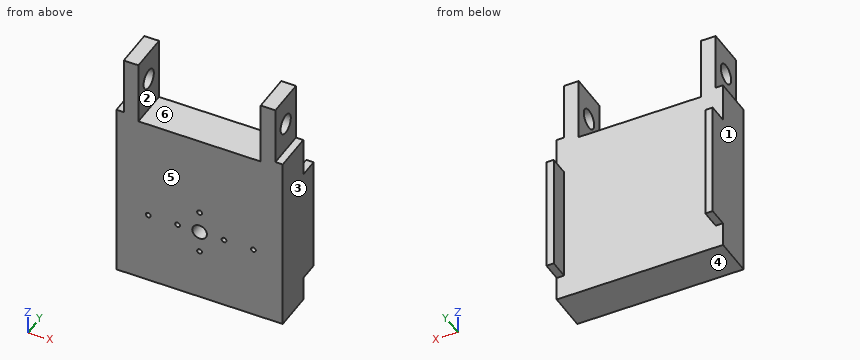
from build123d import *

# Parameters (mm, degrees)
SKETCH_1_W          = 34
SKETCH_1_H          = 49
EXTRUDE_1_DEPTH     = 8
SKETCH_2_W          = 1.5
SKETCH_2_H          = 24
EXTRUDE_2_DEPTH     = 4
SKETCH_3_W          = 1.5
SKETCH_3_H          = 12
SKETCH_3_W_2        = 25
SKETCH_3_H_2        = 13
CUT_EXTRUDE_1_DEPTH = 8
CUT_EXTRUDE_2_REACH = 44.432
SKETCH_4_R          = 2
EXTRUDE_3_DEPTH     = 8
SKETCH_6_R          = 1.5
SKETCH_6_R_2        = 0.5
CUT_EXTRUDE_3_DEPTH = 5
CUT_EXTRUDE_4_DEPTH = 8


with BuildPart() as part:
    # 草图1 → 凸台-拉伸1 (new body)
    with BuildSketch(Plane(origin=(0, 0, 0), x_dir=(1, 0, 0), z_dir=(0, 1, 0))):
        Rectangle(SKETCH_1_W, SKETCH_1_H)
    extrude(amount=EXTRUDE_1_DEPTH)

    # 草图2 → 凸台-拉伸2 (add)
    with BuildSketch(Plane(origin=(0, 8, 0), x_dir=(1, 0, 0), z_dir=(0, 1, 0))):
        with Locations((-16.25, 7.5)):
            Rectangle(SKETCH_2_W, SKETCH_2_H)
        with Locations((16.25, 7.5)):
            Rectangle(SKETCH_2_W, SKETCH_2_H)
    extrude(amount=EXTRUDE_2_DEPTH)

    # 草图3 → 切除-拉伸1 (cut)
    with BuildSketch(Plane(origin=(0, 8, 0), x_dir=(1, 0, 0), z_dir=(0, 1, 0))):
        with Locations((-16.25, -18.5)):
            Rectangle(SKETCH_3_W, SKETCH_3_H)
        with Locations((16.25, -18.5)):
            Rectangle(SKETCH_3_W, SKETCH_3_H)
        with Locations((0, -18)):
            Rectangle(SKETCH_3_W_2, SKETCH_3_H_2)
    extrude(amount=-CUT_EXTRUDE_1_DEPTH, mode=Mode.SUBTRACT)

    # 切除-拉伸2: up to this face of the body (flat: up to its plane)
    cut_extrude_2_end = Plane(part.part.faces().sort_by_distance((15.5, 4, 18.5))[0])
    # 草图4 → 切除-拉伸2 (cut, up to the picked face)
    with BuildSketch(Plane.ZY.offset(15.5), mode=Mode.PRIVATE) as cut_extrude_2_sk1:
        with Locations((18.5, 4)):
            Circle(SKETCH_4_R)
    cut_extrude_2_tool1 = split(extrude(cut_extrude_2_sk1.sketch, amount=-CUT_EXTRUDE_2_REACH, mode=Mode.PRIVATE), bisect_by=cut_extrude_2_end, keep=Keep.BOTH, mode=Mode.PRIVATE)
    add(cut_extrude_2_tool1.solids().sort_by(Axis((-15.5, 4, 18.5), (1, 0, 0)))[0], mode=Mode.SUBTRACT)

    # 草图5 → 凸台-拉伸3 (add)
    with BuildSketch(Plane.XZ):
        Polygon((4, 11.5), (-4, 11.5), (-4, 41.5), (-13, 41.5), (-13, 56.5), (13, 56.5), (13, 41.5), (4, 41.5), align=None)
    extrude(amount=-EXTRUDE_3_DEPTH)

    # 草图6 → 切除-拉伸3 (cut)
    with BuildSketch(Plane.XZ):
        with Locations(Location((0, -9.5, 0), (0, 0, 270))):
            Circle(SKETCH_6_R)
        with Locations(Location((5, -9.5, 0), (0, 0, 270))):
            Circle(SKETCH_6_R_2)
        with Locations(Location((11, -9.5, 0), (0, 0, 270))):
            Circle(SKETCH_6_R_2)
        with Locations(Location((-4.5, -9.5, 0), (0, 0, 270))):
            Circle(SKETCH_6_R_2)
        with Locations(Location((-10.5, -9.5, 0), (0, 0, 270))):
            Circle(SKETCH_6_R_2)
        with Locations(Location((0, -14, 0), (0, 0, 270))):
            Circle(SKETCH_6_R_2)
        with Locations(Location((0, -5, 0), (0, 0, 270))):
            Circle(SKETCH_6_R_2)
    extrude(amount=-CUT_EXTRUDE_3_DEPTH, mode=Mode.SUBTRACT)

    # 草图5<2> → 切除-拉伸4 (cut)
    with BuildSketch(Plane.XZ):
        Polygon((4, 11.5), (-4, 11.5), (-4, 41.5), (-13, 41.5), (-13, 56.5), (13, 56.5), (13, 41.5), (4, 41.5), align=None)
    extrude(amount=-CUT_EXTRUDE_4_DEPTH, mode=Mode.SUBTRACT)


solid = part.part
Can you work these out from the model? Positions are in its coordinate system, mm. Face numbers are marked on the shaded views. A direction names the side the tool comes from. Coordinates: 2 decimals unless noted, no trailing zeros. Loops run counter-clockwise (first coordinate to the right, second up) from the corner with the lowest first, then second, coordinate; pieces in that order, holes last. Notation, with made-up numbers: M 27,87.25 L 73,87.25 A33 cw 73,126.25 Z; hole C 73.5,43.5 d11. An arc over 180 degrees is marked long. Return JSON: item names as keys, results as strings. Group by question number.
Item 1: Imagine slicing it at B-B (y = 9.5). Please give me the cut outline in (x, z), and give its area (3 significant figures).
Item 2: Imagine slicing it at A-A (z = 18.5). Please give me the cut outline in (x, y), and give its area (3 significant figures).
Item 3: On a 3-axis mill with a long thin cutter (end or side, diameter ignored), from which of +Z, -Z, +X, -X, +Y, -Y can I reach the whole of each face in a straight line? I mean the marked faces 5 and 6. Say none if no direction works.
Item 4: I'm going to push flat-ended pins straight in: pin 1 Ø0.8 at (x, y) = (16.5, 10) entering from -Z; pin 2 Ø0.8 at (x, z) = (0, -14) entering from -Y; pin 3 Ø3 at (x, y) = (6.5, 8) entering from +Z; pin 4 Ø1 at (x, y) = (-10.5, 9) entering from +Z. Where does each tip first touch, or does it pass through?
Item 5: Imagine slicing it at D-D (z = -12.5). Please give me the cut outline in (x, y), and give its area (3 significant figures).
Item 6: If I drill on L1, parallel to X at y = 3.6, z = -9.5; L2, parallel to X at y = 2.4, z = -14; L3, parallel to Z at x = -9, y = 5, over which ranges is the centre line in solid material (lowest first)? Write a range as from..to.
Item 7: Thinking about a two-plate mould opening in X: for the marked faces 1, 2, 3 and 4, which applies, released by +X, released by -X, zero draft, split by the parting line, or undercut?
Item 8: Imagine slicing it at C-C (x = 5). Please give me the cut outline in (y, z).
Verdict:
{
 "1": {"outline": "M -17,-19.5 L -15.5,-19.5 L -15.5,4.5 L -17,4.5 Z; M 15.5,-19.5 L 17,-19.5 L 17,4.5 L 15.5,4.5 Z", "area": "72.0 mm^2"},
 "2": {"outline": "M -15.5,0 L -12.5,0 L -12.5,2 L -15.5,2 Z; M -15.5,6 L -12.5,6 L -12.5,8 L -15.5,8 Z; M 12.5,0 L 15.5,0 L 15.5,2 L 12.5,2 Z; M 12.5,6 L 15.5,6 L 15.5,8 L 12.5,8 Z", "area": "24.0 mm^2"},
 "3": {"face 5": "+Z, -Z, +X, -X, -Y", "face 6": "+Z, +Y, -Y"},
 "4": {"pin 1": "stops at z = -19.5", "pin 2": "stops at y = 5", "pin 3": "stops at z = 11.5", "pin 4": "passes through"},
 "5": {"outline": "M -17,0 L 17,0 L 17,12 L 15.5,12 L 15.5,8 L -15.5,8 L -15.5,12 L -17,12 Z", "area": "284 mm^2"},
 "6": {"L1": "x = -17..-11, -10..-5, -4..-1.5, 1.5..4.5, 5.5..10.5, 11.5..17", "L2": "x = -17..-0.5, 0.5..17", "L3": "z = -24.5..11.5"},
 "7": {"face 1": "released by -X", "face 2": "undercut", "face 3": "released by +X", "face 4": "zero draft"},
 "8": {"outline": "M 0,-24.5 L 8,-24.5 L 8,11.5 L 0,11.5 L 0,-9 L 5,-9 L 5,-10 L 0,-10 Z"}
}
